from build123d import *

# Parameters (mm, degrees)
SKETCH1_R           = 17.526
BOSS_EXTRUDE1_DEPTH = 3.175
CUT_EXTRUDE2_DEPTH  = 4.572
CUT_EXTRUDE3_DEPTH  = 4.064


with BuildPart() as part:
    # Sketch1 → Boss-Extrude1 (new body)
    with BuildSketch(Plane(origin=(0, 0, 0), x_dir=(1, 0, 0), z_dir=(0, 1, 0))):
        Circle(SKETCH1_R)
    extrude(amount=-BOSS_EXTRUDE1_DEPTH)

    # Sketch2 → Revolve2 (revolve)
    with BuildSketch(Plane.XY):
        with BuildLine():
            Line((-17.526, -3.175), (0, -3.175))
            Line((0, -3.175), (0, -4.7625))
            ThreePointArc((0, -4.7625), (-8.802377367, -4.403476128), (-17.526, -3.175))
        make_face()
    revolve(axis=Axis((0, 7.394642586, 0), (0, -1, 0)))

    # Sketch4 → Cut-Extrude2 (cut)
    with BuildSketch(Plane(origin=(0, 0, 0), x_dir=(1, 0, 0), z_dir=(0, 1, 0))):
        with BuildLine():
            Line((4.128730565, 9.60699682), (3.175, 7.9375))
            Line((3.175, 7.9375), (-3.175, 7.9375))
            Line((-3.175, 7.9375), (-4.128730565, 9.60699682))
            ThreePointArc((-4.128730565, 9.60699682), (-4.127101881, 10.081811553), (-3.715626661, 10.31875))
            Line((-3.715626661, 10.31875), (3.715626661, 10.31875))
            ThreePointArc((3.715626661, 10.31875), (4.127101881, 10.081811553), (4.128730565, 9.60699682))
        make_face()
    extrude(amount=-CUT_EXTRUDE2_DEPTH, mode=Mode.SUBTRACT)

    # Sketch4_4 → Cut-Extrude3 (cut)
    with BuildSketch(Plane(origin=(0, 0, 0), x_dir=(1, 0, 0), z_dir=(0, 1, 0))):
        Polygon((-3.175, 7.9375), (3.175, 7.9375), (6.35, 7.9375), (6.35, 6.35), (-6.35, 6.35), (-6.35, 7.9375), align=None)
    extrude(amount=-CUT_EXTRUDE3_DEPTH, mode=Mode.SUBTRACT)


solid = part.part
CAD build for the part. Positions are in the model's coordinates, mm. A direction names the side the tool comes from. Round coordinates to 2 decimals unless told otherwise and drop trailing zeros. Put each result on its own line as item: value.
1. 3-axis set-ups, long thin cutter, end or side, ignore diameter. For faces 4 (the flat face through (5, -2, -7.938)), 5 (the flat face through (3.659, -2.182, -8.784)): which of +Z, -Z, +X, -X, +Y, -Y reach the whole face in a straight line?
Geometry check:
face 4: +Y
face 5: +Y, -Y
2. Wall check: line 1 (Y direction, x = -10, z = -4.5); line 2 (Z direction, x = 3.5, y = -1.1); line 3 (Z direction, x = -2.5, y = -0.3). Give the ranges that are in metal, low to high.
Geometry check:
line 1: -4.18 to 0
line 2: -17.17 to -10.32, -8.51 to -7.94, -6.35 to 17.17
line 3: -17.35 to -10.32, -6.35 to 17.35
3. Two-plate mould, pull along Z, no slides. Class faces 1 (the flat face through (0, 0, 0)), 2 (the flat face through (0, -2, -6.35)), 3 (the cylindrical face through (16.72, -1.57, -5.26)): released by +Z, released by -Z, zero draft, split by the parting line, or undercut.
Geometry check:
face 1: zero draft
face 2: undercut
face 3: split by the parting line
4. Pin check, flat tips, straight feed: P1, Ø1.6, axis at x = 4, y = -1, coming from the +Z side; P2, Ø2, axis at x = -10.5, y = -4, coming from the +Z side; P3, Ø1.7, axis at y = -2, z = -7, coming from the -X side. Stop position of each tip, or through.
Geometry check:
P1: z = 17.23
P2: z = 14.44
P3: x = -16.41
